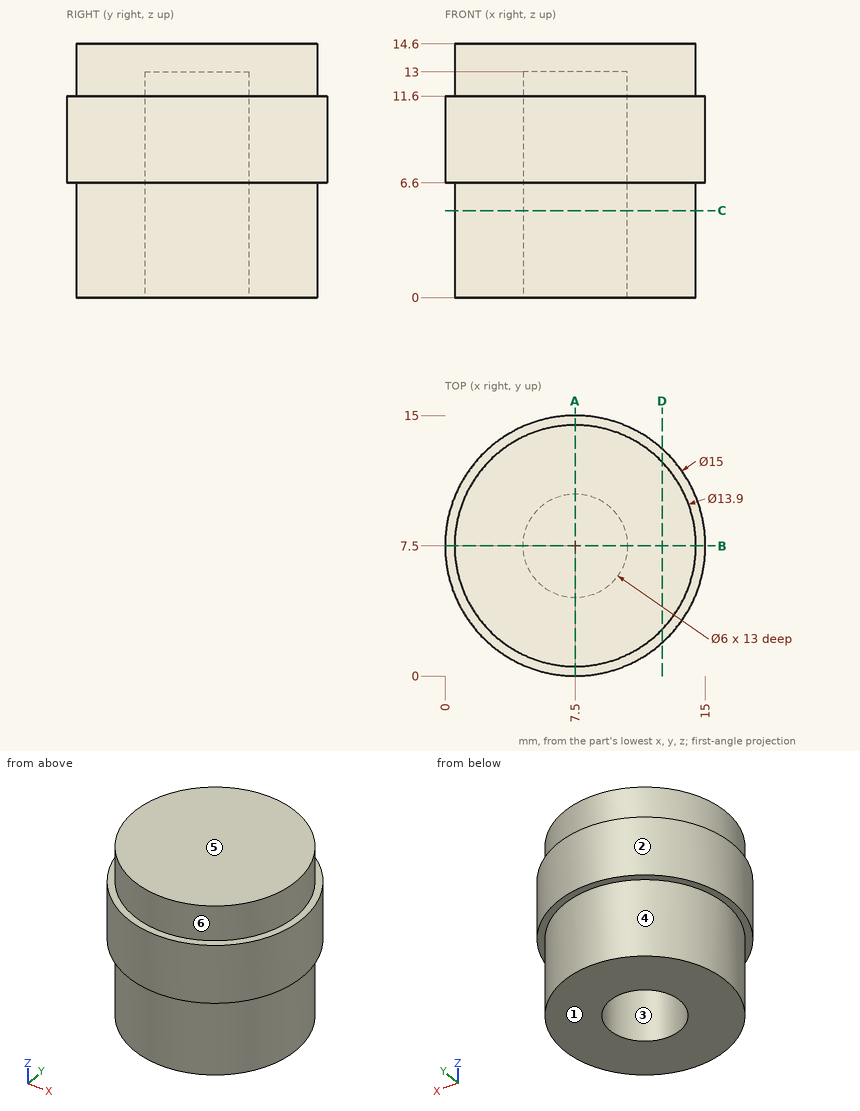
Print and shaded views of the part. All mm, measured from the part's lowest x, y and z. A direction names the side the tool comes from. Give positions to 0.01 mm unless a question says otherwise; leave off trailing zeros. Write each loop counter-clockwise with the first axis right and the second up, starting at its lowest first coordinate (ties: lowest second). Pieces come first, ordered by that corner, then holes. Notation, with made-up numbers: (72.5, 85.25) - (77.5, 85.25) arc R8 ccw to (77.5, 91.25) - close; hole circle Ø5 at (16, 45). An arc over 180 degrees is marked (long way). Put each result on its own line as item: value.
(1) Saw through at D-D (x = 12.5). List the corners of the cut face in (y, z), then the cut area to 3 significant figures.
Working result:
outline: (1.91, 6.6) - (2.67, 6.6) - (2.67, 0) - (12.33, 0) - (12.33, 6.6) - (13.09, 6.6) - (13.09, 11.6) - (12.33, 11.6) - (12.33, 14.6) - (2.67, 14.6) - (2.67, 11.6) - (1.91, 11.6) - close
area: 149 mm^2
(2) Saw through at A-A (x = 7.5). List the corners of the cut face in (y, z).
Working result:
outline: (0, 6.6) - (0.55, 6.6) - (0.55, 0) - (4.5, 0) - (4.5, 13) - (10.5, 13) - (10.5, 0) - (14.45, 0) - (14.45, 6.6) - (15, 6.6) - (15, 11.6) - (14.45, 11.6) - (14.45, 14.6) - (0.55, 14.6) - (0.55, 11.6) - (0, 11.6) - close
(3) Wall check: L1, parallel to Y at x = 7.5, z = 7.75; L2, parallel to Y at x = 7.5, z = 4.5; L3, parallel to Z at x = 7.5, y = 9.75. Give the ranges that are in metal, low to high.
Working result:
L1: 0 to 4.5, 10.5 to 15
L2: 0.55 to 4.5, 10.5 to 14.45
L3: 13 to 14.6
(4) Tool access for the marked faces 4, 5 and 6: list every direction of +Z, -Z, +X, -X, +Y, -Y with a clear straight run to the whole face (end or side of a thin tool).
Working result:
face 4: -Z
face 5: +Z, +X, -X, +Y, -Y
face 6: +Z
(5) Pull direction Y, two halves, no side cores. Call the marked faces 1, 2 and 3: released by +Y, released by -Y, zero draft, split by the parting line, or undercut.
Working result:
face 1: zero draft
face 2: split by the parting line
face 3: undercut
(6) Saw through at C-C (z = 5). List the corners of the cut face in (x, y).
Working result:
outline: circle Ø13.9 at (7.5, 7.5); hole circle Ø6 at (7.5, 7.5)
(7) Drop flat-ended pins along their axis: pin 1 Ø5 at (x, z) = (8, 5.5) entering from -Y; pin 2 Ø1.5 at (x, z) = (12, 11) entering from +Y; pin 3 Ø5 at (x, y) = (7.5, 7.5) entering from -Z; pin 4 Ø1 at (x, z) = (1.5, 2.5) entering from +Y. Give the stop position or say it passes through.
Working result:
pin 1: y = 0
pin 2: y = 14
pin 3: z = 13
pin 4: y = 11.75
